```python
from build123d import *

# Parameters (mm, degrees)
SKETCH_1_W          = 10
SKETCH_1_H          = 4.45
EXTRUDE_1_DEPTH     = 8.9
SKETCH_2_R          = 1.5
EXTRUDE_2_DEPTH     = 1
CUT_EXTRUDE_1_REACH = 15.571
SKETCH_4_W          = 0.254
SKETCH_4_H          = 3.58
SKETCH_3_R          = 0.25
EXTRUDE_3_DEPTH     = 3


# Read off the part's stored shape, not the designer's step: 圆顶1, 圆顶2
with BuildPart() as part:
    # 草图1 → 凸台-拉伸1 (new body)
    with BuildSketch(Plane(origin=(0, 0, 0), x_dir=(1, 0, 0), z_dir=(0, 1, 0))):
        with Locations((5, 0)):
            Rectangle(SKETCH_1_W, SKETCH_1_H)
    extrude(amount=EXTRUDE_1_DEPTH)

    # 草图2 → 凸台-拉伸2 (add)
    with BuildSketch(Plane.XZ):
        with Locations(Location((7.54, 0, 0), (0, 0, 270))):
            Circle(SKETCH_2_R)
        with Locations(Location((2.46, 0, 0), (0, 0, 270))):
            Circle(SKETCH_2_R)
    extrude(amount=EXTRUDE_2_DEPTH)

    # 圆顶1 outline → 圆顶1 (revolve)
    with BuildSketch(Plane(origin=(7.54, 0, 0), x_dir=(1, 0, 0), z_dir=(0, 0, 1))):
        with BuildLine():
            Line((0, -0.999999998), (0, -2.5))
            ThreePointArc((0, -2.5), (1.060660172, -2.060660171), (1.5, -0.999999998))
            Line((1.5, -0.999999998), (0, -0.999999998))
        make_face()
    revolve(axis=Axis((7.54, 0, 0), (0, 1, 0)))

    # 圆顶2 outline → 圆顶2 (revolve)
    with BuildSketch(Plane(origin=(2.46, 0, 0), x_dir=(1, 0, 0), z_dir=(0, 0, 1))):
        with BuildLine():
            Line((0, -0.999999998), (0, -2.5))
            ThreePointArc((0, -2.5), (1.060660172, -2.060660171), (1.5, -0.999999998))
            Line((1.5, -0.999999998), (0, -0.999999998))
        make_face()
    revolve(axis=Axis((2.46, 0, 0), (0, 1, 0)))

    # 草图4 → 切除-拉伸1 (cut, up to next)
    with BuildSketch(Plane.XZ, mode=Mode.PRIVATE) as cut_extrude_1_sk1:
        with Locations((0.127, 0)):
            Rectangle(SKETCH_4_W, SKETCH_4_H)
    cut_extrude_1_tool1 = extrude(cut_extrude_1_sk1.sketch, amount=-CUT_EXTRUDE_1_REACH, mode=Mode.PRIVATE) & part.part
    add(cut_extrude_1_tool1.solids().sort_by_distance((0.127, 0, 0))[0], mode=Mode.SUBTRACT)

    # 草图3 → 凸台-拉伸3 (add)
    with BuildSketch(Plane.ZY.offset(-0.254)):
        with Locations(Location((-1.27, 5.08, 0), (0, 0, 180))):
            Circle(SKETCH_3_R)
        with Locations(Location((-1.27, 7.62, 0), (0, 0, 180))):
            Circle(SKETCH_3_R)
        with Locations(Location((1.27, 7.62, 0), (0, 0, 180))):
            Circle(SKETCH_3_R)
        with Locations(Location((1.27, 5.08, 0), (0, 0, 180))):
            Circle(SKETCH_3_R)
    extrude(amount=EXTRUDE_3_DEPTH)


solid = part.part
```
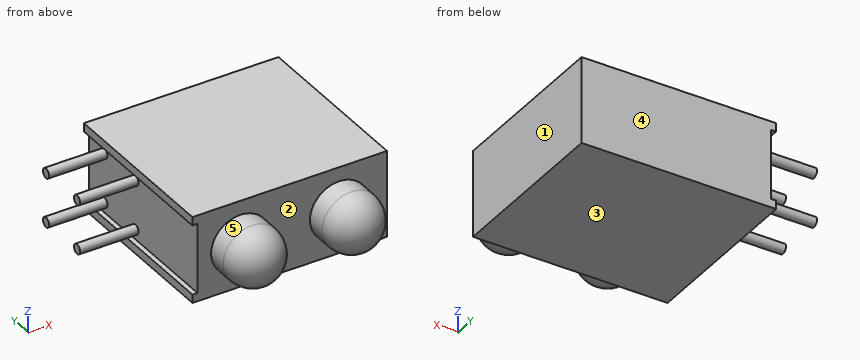
The model under review builds one solid part; all positions refer to its coordinate system, in mm. Face numbers are marked on the shaded views. A direction names the side the tool comes from. Round coordinates to 2 decimals unless told otherwise and drop trailing zeros. Order: outer loops, then holes, each group sorted by start corner. A loop starts at its lowest first (then second) coordinate and runs counter-clockwise, first axis right, second up.
(1) Take a section at A-A, the plane x = 2.46. State the section outline as (y, z) points (3 decimals).
Working result:
outline: (-1, -1.5) - (0, -1.5) - (0, -2.225) - (8.9, -2.225) - (8.9, 2.225) - (0, 2.225) - (0, 1.5) - (-1, 1.5) arc R1.5 ccw to start
(2) Take a section at C-C, the plane y = 5.08. State the section outline as (x, z) points (3 decimals).
Working result:
outline: (-2.746, -1.52) - (0.254, -1.52) - (0.254, -1.79) - (0, -1.79) - (0, -2.225) - (10, -2.225) - (10, 2.225) - (0, 2.225) - (0, 1.79) - (0.254, 1.79) - (0.254, 1.52) - (-2.746, 1.52) - (-2.746, 1.02) - (0.254, 1.02) - (0.254, -1.02) - (-2.746, -1.02) - close
(3) Wall thickness on L1, parallel to X at y = 1.75, z = -0.7; L2, parallel to Y at x = 8.5, z = -2; L3, parallel to X at y = 4, z = 1.95: over which ranges is each line inside the solid? List them lowest first.
Working result:
L1: x = 0.25 to 10
L2: y = 0 to 8.9
L3: x = 0 to 10
(4) Take a section at B-B, the plane z = 0. State the section outline as (x, y) points, plus the area to 3 significant figures.
Working result:
outline: (0.25, 0) - (0.96, 0) - (0.96, -1) arc R1.5 ccw to (3.96, -1) - (3.96, 0) - (6.04, 0) - (6.04, -1) arc R1.5 ccw to (9.04, -1) - (9.04, 0) - (10, 0) - (10, 8.9) - (0.25, 8.9) - close
area: 99.8 mm2
(5) Tool access review of the marked faces 4 and 5: name each direction out of +Z, -Z, +X, -X, +Y, -Y from which nothing blocks a thin tool from reaching the whole face with its end or side.
Working result:
face 4: +Z, -Z, +X, -X, +Y
face 5: -Y
(6) For P1, Ø0.5, axis at y = 4, z = 2, coming from the -X side, flat-tipped, find the tip position at first contact; note if it passes through.
Working result:
P1: stops at x = 0
(7) Mouldability with a two-part tool opening along X and no side actions: class the marked faces 1, 2 and 3 as released by +X, released by -X, zero draft, split by the parting line, or undercut.
Working result:
face 1: released by +X
face 2: undercut
face 3: zero draft
(8) Take a section at D-D, the plane y = 0.75. State the section outline as (x, z) points (3 decimals), plus the area to 3 significant figures.
Working result:
outline: (0, -2.225) - (10, -2.225) - (10, 2.225) - (0, 2.225) - (0, 1.79) - (0.254, 1.79) - (0.254, -1.79) - (0, -1.79) - close
area: 43.6 mm2
